Study the drawing (mm; zero at the part's minimum x, y, z) and answer. A direction names the side the tool comes from. Give positions to 0.01 mm unless a question says otherwise; leave off trailing zeros. Loops run counter-clockwise (first coordinate to the right, second up) from the corner with the lowest first, then second, coordinate; pieces in that order, holes last. Notation, with made-up numbers: (73, 22.25) -> (120, 22.25) arc R18 ccw to (120, 53.25) -> close; hole circle Ø3 at (50, 65.5). An arc over 180 degrees is marked (long way). One line per question, with ' | ' between items. Start each with the question number.
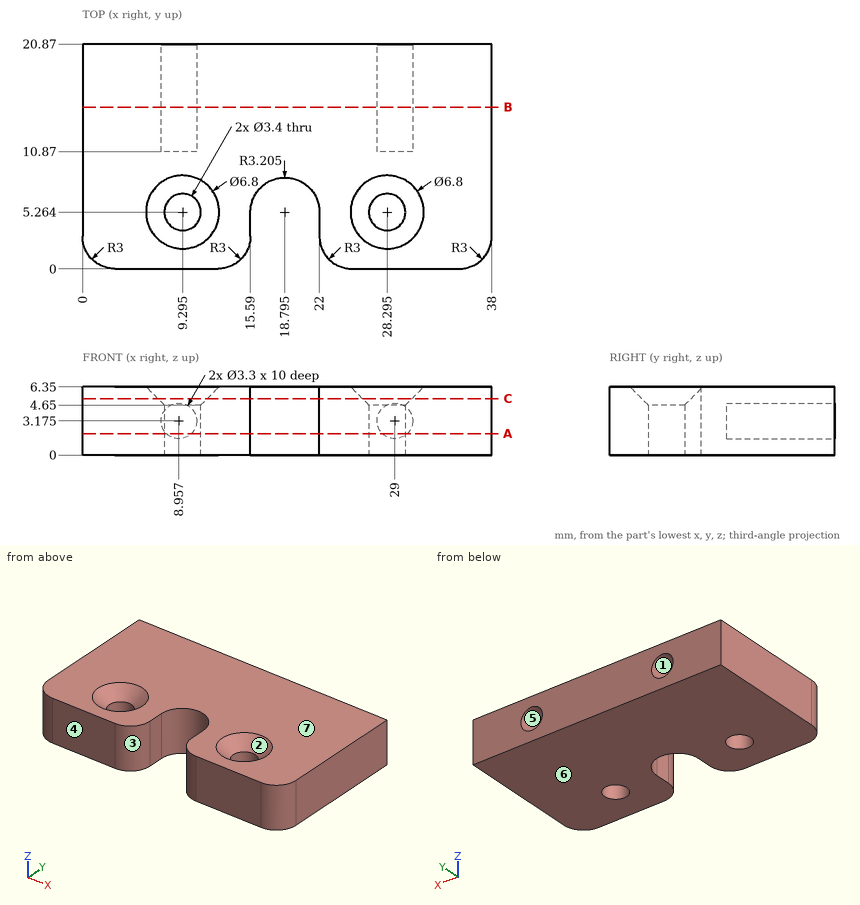
1. Straight lines are drawn through the part: L1, parallel to X at y = 3.5, z = 2.5; L2, parallel to X at y = 19.25, z = 4.25 (1 decimal); L3, parallel to X at y = 16.5, z = 2 (1 decimal). For each, find the intervals that lie inside material, in ascending order.
2. The part is cut by section B-B (y = 15). Count the separate pieces of the cut face and the enclosed holes in it, plus the area to 3 significant figures.
3. Determine the mould class of the marked faces 4, 5, 6 and 7 for opening direction Z: released by +Z, released by -Z, zero draft, split by the parting line, or undercut.
4. Each of these flat-tipped pins is pushed along its axis until it touches: pin 1 Ø5.5 at (x, y) = (28.3, 5.26) entering from +Z; pin 2 Ø4 at (x, y) = (19, 4.5) entering from -Z; pin 3 Ø1 at (x, z) = (9.5, 3.5) entering from +Y. Where does it stop, or does it pass through?
5. The part is cut by section A-A (z = 2). Write down the section's boundary in (x, y) (1 decimal), plus the area to 3 significant figures.
6. For the marked faces 1, 2 and 3, determine the directions among +Z, -Z, +X, -X, +Y, -Y from which every point of the face is accessible in a straight line to the end or side of a thin tool.
7. The part is cut by section C-C (z = 5.25). Write down the section's boundary in (x, y) (1 decimal).
Check sheet entries:
1) L1: x = 0 to 15.59, 22 to 38 | L2: x = 0 to 7.7, 10.2 to 27.7, 30.3 to 38 | L3: x = 0 to 7.8, 10.1 to 27.8, 30.2 to 38
2) separate pieces: 1 | enclosed holes: 2 | area: 224 mm^2
3) face 4: zero draft | face 5: undercut | face 6: released by -Z | face 7: released by +Z
4) pin 1: stops at z = 5.71 | pin 2: passes through | pin 3: stops at y = 10.87
5) outline: (0, 3) arc R3 ccw to (3, 0) -> (12.6, 0) arc R3 ccw to (15.6, 3) -> (15.6, 5.3) arc R3.2 cw to (22, 5.3) -> (22, 3) arc R3 ccw to (25, 0) -> (35, 0) arc R3 ccw to (38, 3) -> (38, 20.9) -> (30.2, 20.9) -> (30.2, 10.9) -> (27.8, 10.9) -> (27.8, 20.9) -> (10.1, 20.9) -> (10.1, 10.9) -> (7.8, 10.9) -> (7.8, 20.9) -> (0, 20.9) -> close; hole circle Ø3.4 at (9.3, 5.3); hole circle Ø3.4 at (28.3, 5.3) | area: 671 mm^2
6) face 1: +Y | face 2: +Z | face 3: +Z, -Z, -Y
7) outline: (0, 3) arc R3 ccw to (3, 0) -> (12.6, 0) arc R3 ccw to (15.6, 3) -> (15.6, 5.3) arc R3.2 cw to (22, 5.3) -> (22, 3) arc R3 ccw to (25, 0) -> (35, 0) arc R3 ccw to (38, 3) -> (38, 20.9) -> (0, 20.9) -> close; hole circle Ø4.6 at (9.3, 5.3); hole circle Ø4.6 at (28.3, 5.3)
